The listing builds one solid part. Answer for the finished solid, in the listing's coordinates (mm). Give positions to 0.01 mm unless a question says otherwise; leave off trailing zeros. Loops run counter-clockwise (first coordinate to the right, second up) from the corner with the lowest first, then second, coordinate; pieces in that order, holes last. Notation, with made-up numbers: (47, 24) - (92, 24) arc R19 ccw to (92, 44) - close; hole circle Ø9 at (34, 58.5). An arc over 180 degrees is marked (long way). Write item = value, one per line. Start each with the question number.
1) The part is cut by section C-C on y = 95. Write down the section's boundary in (x, z), plus the area to 3 significant figures.
2) The part is cut by section B-B on z = 0.8. State how many separate pieces and enclosed holes the cut face has, plus the area to 3 significant figures.
3) Flat-ended cylindrical pins translate along their axes: P1, Ø1.8, axis at x = 78.17, y = -136.31, coming from the -Z side; P2, Ø4.5, axis at x = 41.59, y = 136.21, coming from the -Z side; P3, Ø1, axis at x = -76, z = 4, coming from the -Y side; P4, Ø1.5, axis at y = 111, z = 1.5, coming from the -X side. Find the tip coordinate at first contact, or state that the pin passes through.
4) Consider probe 1 along Y at (x, z) = (-31.5, 1.25); probe 2 along X at (y, z) = (-57, 1.8); probe 3 along Y at (x, z) = (-111, 2.6). Determine where each line is inside the solid, lowest interval first.
5) The part is cut by section A-A on y = -49. Write down the section's boundary in (x, z).
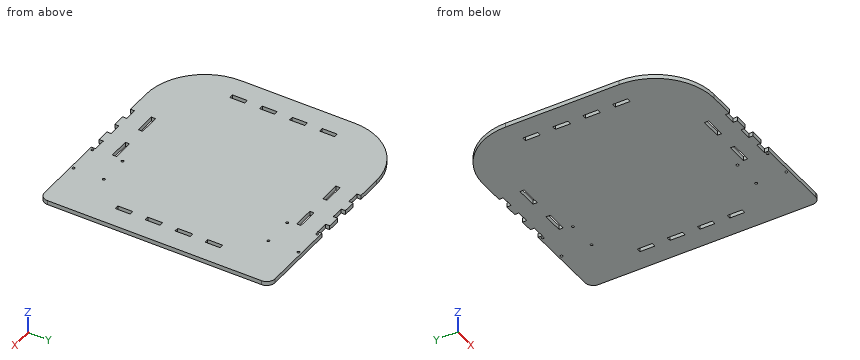
from build123d import *

# Parameters (mm, degrees)
SKETCH1_W           = 279.4
SKETCH1_H           = 279.4
BOSS_EXTRUDE1_DEPTH = 5.08
FILLET1_R           = 70.96
FILLET2_R           = 70.960000066
FILLET3_R           = 10
FILLET4_R           = 10
SKETCH2_W           = 25.4
SKETCH2_H           = 5.08
CUT_EXTRUDE1_DEPTH  = 7.62
SKETCH3_W           = 15.24
SKETCH3_H           = 5.08
CUT_EXTRUDE2_DEPTH  = 5.08
SKETCH4_W           = 25.4
SKETCH4_H           = 5.08
SKETCH4_W_2         = 15.24
CUT_EXTRUDE3_DEPTH  = 5.08
SKETCH5_W           = 5.08
SKETCH5_H           = 18.142857143
CUT_EXTRUDE4_DEPTH  = 5.08
SKETCH9_R           = 1.521747373
SKETCH9_R_2         = 1.52437788
SKETCH9_R_3         = 1.483080804
SKETCH9_R_4         = 1.509853377
CUT_EXTRUDE5_DEPTH  = 5.08
SKETCH10_R          = 1.496375704
SKETCH10_R_2        = 1.496038234
SKETCH10_R_3        = 1.499292219
SKETCH10_R_4        = 1.440705467
CUT_EXTRUDE6_DEPTH  = 5.08


with BuildPart() as part:
    # Sketch1 → Boss-Extrude1 (new body)
    with BuildSketch(Plane.XY):
        Rectangle(SKETCH1_W, SKETCH1_H)
    extrude(amount=BOSS_EXTRUDE1_DEPTH)

    # Fillet1
    fillet1_edges = [part.edges().sort_by_distance(p)[0] for p in [
        (-139.7, 139.7, 2.54),
    ]]
    fillet(fillet1_edges, radius=FILLET1_R)

    # Fillet2
    fillet2_edges = [part.edges().sort_by_distance(p)[0] for p in [
        (-139.7, -139.7, 2.54),
    ]]
    fillet(fillet2_edges, radius=FILLET2_R)

    # Fillet3
    fillet3_edges = [part.edges().sort_by_distance(p)[0] for p in [
        (139.7, 139.7, 2.54),
    ]]
    fillet(fillet3_edges, radius=FILLET3_R)

    # Fillet4
    fillet4_edges = [part.edges().sort_by_distance(p)[0] for p in [
        (139.7, -139.7, 2.54),
    ]]
    fillet(fillet4_edges, radius=FILLET4_R)

    # Sketch2 → Cut-Extrude1 (cut)
    with BuildSketch(Plane.XY.offset(5.08)):
        with Locations((-25.4, -111.76)):
            Rectangle(SKETCH2_W, SKETCH2_H)
        with Locations((25.4, -111.76)):
            Rectangle(SKETCH2_W, SKETCH2_H)
    extrude(amount=-CUT_EXTRUDE1_DEPTH, mode=Mode.SUBTRACT)

    # Sketch3 → Cut-Extrude2 (cut)
    with BuildSketch(Plane.XY.offset(5.08)):
        with Locations((-30.48, -137.16)):
            Rectangle(SKETCH3_W, SKETCH3_H)
        with Locations((0, -137.16)):
            Rectangle(SKETCH3_W, SKETCH3_H)
        with Locations((30.48, -137.16)):
            Rectangle(SKETCH3_W, SKETCH3_H)
    extrude(amount=-CUT_EXTRUDE2_DEPTH, mode=Mode.SUBTRACT)

    # Sketch4 → Cut-Extrude3 (cut)
    with BuildSketch(Plane.XY.offset(5.08)):
        with Locations((-25.4, 111.76)):
            Rectangle(SKETCH4_W, SKETCH4_H)
        with Locations((25.4, 111.76)):
            Rectangle(SKETCH4_W, SKETCH4_H)
        with Locations((-30.48, 137.16)):
            Rectangle(SKETCH4_W_2, SKETCH4_H)
        with Locations((0, 137.16)):
            Rectangle(SKETCH4_W_2, SKETCH4_H)
        with Locations((30.48, 137.16)):
            Rectangle(SKETCH4_W_2, SKETCH4_H)
    extrude(amount=-CUT_EXTRUDE3_DEPTH, mode=Mode.SUBTRACT)

    # Sketch5 → Cut-Extrude4 (cut)
    with BuildSketch(Plane(origin=(0, 0, 0), x_dir=(-1, 0, 0), z_dir=(0, 0, -1))):
        with Locations((111.76, -54.428571429)):
            Rectangle(SKETCH5_W, SKETCH5_H)
        with Locations((111.76, -18.142857143)):
            Rectangle(SKETCH5_W, SKETCH5_H)
        with Locations((111.76, 18.142857143)):
            Rectangle(SKETCH5_W, SKETCH5_H)
        with Locations((111.76, 54.428571429)):
            Rectangle(SKETCH5_W, SKETCH5_H)
        with Locations((-111.76, -54.428571429)):
            Rectangle(SKETCH5_W, SKETCH5_H)
        with Locations((-111.76, -18.142857143)):
            Rectangle(SKETCH5_W, SKETCH5_H)
        with Locations((-111.76, 18.142857143)):
            Rectangle(SKETCH5_W, SKETCH5_H)
        with Locations((-111.76, 54.428571429)):
            Rectangle(SKETCH5_W, SKETCH5_H)
    extrude(amount=-CUT_EXTRUDE4_DEPTH, mode=Mode.SUBTRACT)

    # Sketch9 → Cut-Extrude5 (cut)
    with BuildSketch(Plane(origin=(0, 0, 0), x_dir=(-1, 0, 0), z_dir=(0, 0, -1))):
        with Locations((-78.174292247, -99.783948619)):
            Circle(SKETCH9_R)
        with Locations((-41.5890041, -99.783948619)):
            Circle(SKETCH9_R_2)
        with Locations((-41.5890041, -136.30594042)):
            Circle(SKETCH9_R_3)
        with Locations((-78.174292247, -136.30594042)):
            Circle(SKETCH9_R_4)
    extrude(amount=-CUT_EXTRUDE5_DEPTH, mode=Mode.SUBTRACT)

    # Sketch10 → Cut-Extrude6 (cut)
    with BuildSketch(Plane(origin=(0, 0, 0), x_dir=(-1, 0, 0), z_dir=(0, 0, -1))):
        with Locations((-78.112727159, 136.214508439)):
            Circle(SKETCH10_R)
        with Locations((-78.112727159, 99.715329187)):
            Circle(SKETCH10_R_2)
        with Locations((-41.590577287, 99.715329187)):
            Circle(SKETCH10_R_3)
        with Locations((-41.590577287, 136.214508439)):
            Circle(SKETCH10_R_4)
    extrude(amount=-CUT_EXTRUDE6_DEPTH, mode=Mode.SUBTRACT)


solid = part.part
Answer below:
q1.outline = (-134.66, 0) - (139.7, 0) - (139.7, 5.08) - (-134.66, 5.08) - close
q1.area = 1,390 mm2
q2.separate_pieces = 1
q2.enclosed_holes = 20
q2.area = 74,100 mm2
q3.P1 = through
q3.P2 = 0
q3.P3 = -139.38
q3.P4 = -126.29
q4.probe_1 = -134.62 to -114.3, -109.22 to 109.22, 114.3 to 134.62
q4.probe_2 = -139.7 to -114.3, -109.22 to 109.22, 114.3 to 139.7
q4.probe_3 = -125.74 to -63.5, -45.36 to -27.21, -9.07 to 9.07, 27.21 to 45.36, 63.5 to 125.74
q5.outline = (-139.7, 0) - (-114.3, 0) - (-114.3, 5.08) - (-139.7, 5.08) - close; (-109.22, 0) - (109.22, 0) - (109.22, 5.08) - (-109.22, 5.08) - close; (114.3, 0) - (139.7, 0) - (139.7, 5.08) - (114.3, 5.08) - close
